Check sheet for the modelled part. Datum: model origin and axes. Units: mm. A direction names the side the tool comes from. Give positions to 0.01 mm unless a question says otherwise; leave off trailing zeros. Order: outer loops, then holes, each group sorted by start corner. A loop starts at its lowest first (then second) coordinate and runs counter-clockwise, first axis right, second up.
from build123d import *

# Parameters (mm, degrees)
F1_DEPTH = 11.43
F2_W     = 6.35
F2_H     = 5.08
F3_DEPTH = 25.4
F4_R     = 7.62
F5_DEPTH = 66.04
F6_R     = 5.08
F7_DEPTH = 63.5
F8_R     = 1.27


with BuildPart() as f1:
    # F0 (on Right) → F1 (new body, symmetric)
    with BuildSketch(Plane.YZ):
        Polygon((35.56, 12.7), (0, 12.7), (0, 0), (0, -2.54), (35.56, -2.54), (35.56, 0), align=None)
    extrude(amount=F1_DEPTH, both=True)

    # F2 (on face) → F3 (cut)
    with BuildSketch(Plane.XY.offset(12.7)):
        with Locations((-8.255, 2.54)):
            Rectangle(F2_W, F2_H)
        with Locations((8.255, 2.54)):
            Rectangle(F2_W, F2_H)
    extrude(amount=-F3_DEPTH, mode=Mode.SUBTRACT)

    # F4 (on face) → F5 (join)
    with BuildSketch(Plane(origin=(0, 35.56, 0), x_dir=(-1, 0, 0), z_dir=(0, 1, 0))):
        with Locations((0, 5.08)):
            Circle(F4_R)
    extrude(amount=F5_DEPTH)

    # F6 (on face) → F7 (cut)
    with BuildSketch(Plane(origin=(0, 101.6, 0), x_dir=(-1, 0, 0), z_dir=(0, 1, 0))):
        with Locations((0, 5.08)):
            Circle(F6_R)
    extrude(amount=-F7_DEPTH, mode=Mode.SUBTRACT)

    # F8
    f8_edges = [f1.edges().sort_by_distance(p)[0] for p in [
        (-11.43, 20.32, 12.7),
        (11.43, 20.32, 12.7),
    ]]
    fillet(f8_edges, radius=F8_R)


solid = f1.part
1) Section check D-D, the plane z = 1.25. Record the cut outline in (x, y), then the cut area to 3 significant figures.
Recorded:
outline: (-11.43, 5.08) - (-5.08, 5.08) - (-5.08, 0) - (5.08, 0) - (5.08, 5.08) - (11.43, 5.08) - (11.43, 35.56) - (6.59, 35.56) - (6.59, 101.6) - (3.34, 101.6) - (3.34, 38.1) - (-3.34, 38.1) - (-3.34, 101.6) - (-6.59, 101.6) - (-6.59, 35.56) - (-11.43, 35.56) - close
area: 1,190 mm2
2) Set-up check for faces 4 (the face through (1.1, 70.29, 0.12)), 5 (the face through (8, 5.08, 5)), 6 (the face through (-5.08, 3, 5)): record each of +Z, -Z, +X, -X, +Y, -Y from which the full face is reachable in a straight line by a thin tool's end or side.
Recorded:
face 4: +Y
face 5: +Z, -Z, +X, -Y
face 6: +Z, -Z, -X, -Y
3) Section check B-B, the plane z = 5.08. Record the cut outline in (x, y).
Recorded:
outline: (-11.43, 5.08) - (-5.08, 5.08) - (-5.08, 0) - (5.08, 0) - (5.08, 5.08) - (11.43, 5.08) - (11.43, 35.56) - (7.62, 35.56) - (7.62, 101.6) - (5.08, 101.6) - (5.08, 38.1) - (-5.08, 38.1) - (-5.08, 101.6) - (-7.62, 101.6) - (-7.62, 35.56) - (-11.43, 35.56) - close
4) Section check A-A, the plane y = 53. Record the cut outline in (x, z).
Recorded:
outline: circle Ø15.24 at (0, 5.08); hole circle Ø10.16 at (0, 5.08)
5) Material ranges on L1, parallel to Z at x = 0, y = 55; L2, parallel to X at y = 59, z = 5.5; L3, parallel to Y at x = 1.5, z = 1.25, recorded low to high.
Recorded:
L1: z = -2.54 to 0, 10.16 to 12.7
L2: x = -7.61 to -5.06, 5.06 to 7.61
L3: y = 0 to 38.1
6) Section check C-C, the plane x = 2. Record the cut outline in (y, z).
Recorded:
outline: (0, -2.54) - (35.56, -2.54) - (35.56, -2.27) - (101.6, -2.27) - (101.6, 0.41) - (38.1, 0.41) - (38.1, 9.75) - (101.6, 9.75) - (101.6, 12.43) - (35.56, 12.43) - (35.56, 12.7) - (0, 12.7) - close
7) Depth check by flat-ended pin: pin 1 Ø5 at (x, z) = (9, 3) entering from -Y; pin 2 Ø5.5 at (y, z) = (1.5, 3.5) entering from +X; pin 3 Ø5 at (x, z) = (-0.5, 6.5) entering from +Y. Enter the tip coordinate at first touch or a pass-through.
Recorded:
pin 1: stops at y = 5.08
pin 2: stops at x = 5.08
pin 3: stops at y = 38.1
8) Draft check along Z on faces 1 (the face through (-8, 5.08, 5)), 2 (the face through (0, 38.1, 5)), 3 (the face through (0, 18, -2.54)). Enter one of: +Z half, -Z half, draft (parallel to the pull), parting line (faces both ways), or undercut.
Recorded:
face 1: draft
face 2: undercut
face 3: -Z half
